```python
from build123d import *

# Parameters (mm, degrees)
CROQUIS1_R              = 4
SALIENTE_EXTRUIR1_DEPTH = 1.497272789
CROQUIS3_R              = 2.5
CORTAR_EXTRUIR2_DEPTH   = 3
CROQUIS4_R              = 15.8
CORTAR_EXTRUIR3_DEPTH   = 10
CROQUIS5_W              = 12
CROQUIS5_H              = 7.5
CORTAR_EXTRUIR4_DEPTH   = 10
CROQUIS6_R              = 1.600000002
CORTAR_EXTRUIR5_DEPTH   = 10
CROQUIS9_R              = 1.787352587
CROQUIS9_R_2            = 1.8
CROQUIS9_R_3            = 1.832705365
CROQUIS9_R_4            = 1.812354621
CORTAR_EXTRUIR7_DEPTH   = 10
CROQUIS10_R             = 2
CROQUIS10_R_2           = 2.1
CORTAR_EXTRUIR8_DEPTH   = 10


with BuildPart() as part:
    # Croquis1 → Saliente-Extruir1 (new, symmetric)
    with BuildSketch(Plane(origin=(0, 0, 0), x_dir=(1, 0, 0), z_dir=(0, 1, 0))):
        Polygon((-77, -42), (-77, -54), (77, -54), (77, -42), (74, -42), (74, -28), (77, -28), (77, -20), (74, -20), (74, -12), (77, -12), (77, -4), (74, -4), (74, -1.5), (74, 1.5), (74, 4), (77, 4), (77, 12), (74, 12), (74, 14.497912952), (70.25, 14.497912952), (70.25, 12), (67.25, 12), (67.25, 14.497912952), (66.27, 14.497912952), (66.27, 17.992083938), (67.25, 17.992083938), (67.25, 20), (70.25, 20), (70.25, 17.992083938), (74, 17.992083938), (74, 20), (77, 20), (77, 28), (74, 28), (74, 42), (77, 42), (77, 54), (65, 54), (65, 51), (55, 51), (55, 54), (45, 54), (45, 51), (31.5, 51), (31.5, 47.25), (34, 47.25), (34, 44.25), (31.5, 44.25), (31.5, 43.27), (28.5, 43.27), (28.5, 44.25), (26, 44.25), (26, 47.25), (28.5, 47.25), (28.5, 51), (15, 51), (15, 54), (5, 54), (5, 51), (-5, 51), (-5, 54), (-15, 54), (-15, 51), (-28.5, 51), (-28.5, 47.25), (-26, 47.25), (-26, 44.25), (-28.5, 44.25), (-28.5, 43.27), (-31.5, 43.27), (-31.5, 44.25), (-34, 44.25), (-34, 47.25), (-31.5, 47.25), (-31.5, 51), (-45, 51), (-45, 54), (-55, 54), (-55, 51), (-65, 51), (-65, 54), (-77, 54), (-77, 42), (-74, 42), (-74, 28), (-77, 28), (-77, 20), (-74, 20), (-74, 17.992083938), (-70.25, 17.992083938), (-70.25, 20), (-67.25, 20), (-67.25, 17.992083938), (-66.27, 17.992083938), (-66.27, 14.497912952), (-67.25, 14.497912952), (-67.25, 12), (-70.25, 12), (-70.25, 14.497912952), (-74, 14.497912952), (-74, 12), (-77, 12), (-77, 4), (-74, 4), (-74, 1.5), (-74, -1.5), (-74, -4), (-77, -4), (-77, -12), (-74, -12), (-74, -20), (-77, -20), (-77, -28), (-74, -28), (-74, -42), align=None)
        with Locations(Location((-65, -48, 0), (0, 0, 270))):
            Circle(CROQUIS1_R, mode=Mode.SUBTRACT)
        with BuildLine():
            Line((55, -49.6), (53, -49.6))
            ThreePointArc((53, -49.6), (52.646446609, -49.453553391), (52.5, -49.1))
            Line((52.5, -49.1), (52.5, -46.4))
            Line((52.5, -46.4), (55.5, -46.4))
            Line((55.5, -46.4), (55.5, -49.1))
            ThreePointArc((55.5, -49.1), (55.353553391, -49.453553391), (55, -49.6))
        make_face(mode=Mode.SUBTRACT)
    extrude(amount=SALIENTE_EXTRUIR1_DEPTH, both=True)

    # Croquis3 → Cortar-Extruir2 (cut)
    with BuildSketch(Plane(origin=(0, 1.497272789, 0), x_dir=(1, 0, 0), z_dir=(0, 1, 0))):
        with Locations(Location((-19.5, 33.79, 0), (0, 0, 270))):
            Circle(CROQUIS3_R)
        with Locations(Location((19.5, 33.79, 0), (0, 0, 270))):
            Circle(CROQUIS3_R)
    extrude(amount=-CORTAR_EXTRUIR2_DEPTH, mode=Mode.SUBTRACT)

    # Croquis4 → Cortar-Extruir3 (cut)
    with BuildSketch(Plane.XZ.offset(1.497272789)):
        with Locations(Location((0, -33.79, 0), (0, 0, 270))):
            Circle(CROQUIS4_R)
    extrude(amount=-CORTAR_EXTRUIR3_DEPTH, mode=Mode.SUBTRACT)

    # Croquis5 → Cortar-Extruir4 (cut)
    with BuildSketch(Plane.XZ.offset(1.497272789)):
        with Locations((-33.25, -35.6)):
            Rectangle(CROQUIS5_W, CROQUIS5_H)
        with Locations((33.25, -35.6)):
            Rectangle(CROQUIS5_W, CROQUIS5_H)
    extrude(amount=-CORTAR_EXTRUIR4_DEPTH, mode=Mode.SUBTRACT)

    # Croquis6 → Cortar-Extruir5 (cut)
    with BuildSketch(Plane(origin=(0, 1.497272789, 0), x_dir=(1, 0, 0), z_dir=(0, 1, 0))):
        with Locations(Location((33.25, 13.2, 0), (0, 0, 270))):
            Circle(CROQUIS6_R)
        with Locations(Location((-33.25, 13.2, 0), (0, 0, 270))):
            Circle(CROQUIS6_R)
    extrude(amount=-CORTAR_EXTRUIR5_DEPTH, mode=Mode.SUBTRACT)

    # Croquis9 → Cortar-Extruir7 (cut)
    with BuildSketch(Plane(origin=(0, 1.497272789, 0), x_dir=(1, 0, 0), z_dir=(0, 1, 0))):
        with Locations(Location((69.85, 46.119647413, 0), (0, 0, 270))):
            Circle(CROQUIS9_R)
        with Locations(Location((69.8, 27.693127607, 0), (0, 0, 270))):
            Circle(CROQUIS9_R_2)
        with Locations(Location((69.85, -21.925705365, 0), (0, 0, 270))):
            Circle(CROQUIS9_R_3)
        with Locations(Location((69.8, -40.306872393, 0), (0, 0, 270))):
            Circle(CROQUIS9_R_2)
        with Locations(Location((-69.8, -40.306872393, 0), (0, 0, 270))):
            Circle(CROQUIS9_R_2)
        with Locations(Location((-69.85, -21.925705365, 0), (0, 0, 270))):
            Circle(CROQUIS9_R_3)
        with Locations(Location((-66.4, 27.693127607, 0), (0, 0, 270))):
            Circle(CROQUIS9_R_2)
        with Locations(Location((-66.4, 46.119647413, 0), (0, 0, 270))):
            Circle(CROQUIS9_R_4)
    extrude(amount=-CORTAR_EXTRUIR7_DEPTH, mode=Mode.SUBTRACT)

    # Croquis10 → Cortar-Extruir8 (cut)
    with BuildSketch(Plane(origin=(0, 1.497272789, 0), x_dir=(1, 0, 0), z_dir=(0, 1, 0))):
        with Locations(Location((-19, 4.95, 0), (0, 0, 270))):
            Circle(CROQUIS10_R)
        with Locations(Location((19, 4.95, 0), (0, 0, 270))):
            Circle(CROQUIS10_R_2)
        with Locations(Location((19, -33.05, 0), (0, 0, 270))):
            Circle(CROQUIS10_R_2)
        with Locations(Location((-19, -33.05, 0), (0, 0, 270))):
            Circle(CROQUIS10_R)
    extrude(amount=-CORTAR_EXTRUIR8_DEPTH, mode=Mode.SUBTRACT)


solid = part.part
```
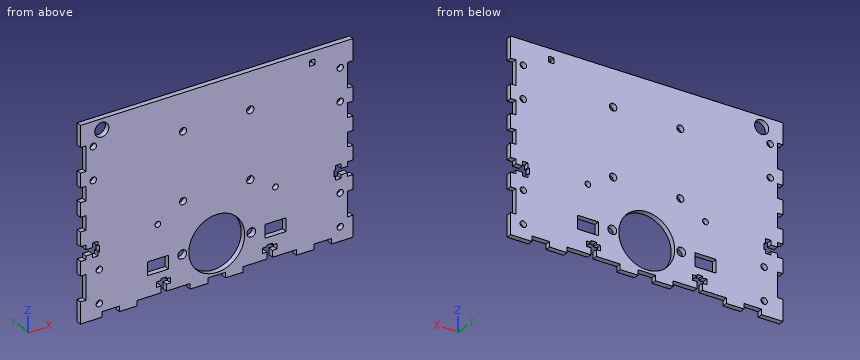
Model file for the job. Use its own axes, mm. Coordinates: 2 decimals unless noted, no trailing zeros. Loops run counter-clockwise (first coordinate to the right, second up) from the corner with the lowest first, then second, coordinate; pieces in that order, holes last. Notation, with made-up numbers: M 36.5,20 L 69.5,20 A22 cw 69.5,42 Z; hole C -9.75,71.5 d11. An arc over 180 degrees is marked long. Use CSV: the item, a comma, the result in double quotes. Start each with the question number.
1. Band-saw the part on A-A, the plane y = -0.1. Give the number of separate pieces and of enclosed holes in the cut face, then the cut area to 3 significant figures.
2. Probe probe 1 along X at (y, z) = (-0.1, -33.79); probe 2 along Z at (x, y) = (70, 1); probe 3 along X at (y, z) = (-0.25, -4.95). List the from-to ranges inside material, lowest first. Write a range as [from, to].
3. Band-saw the part on B-B, the plane x = 62. List the corners of the cut face in (y, z), then the cut area to 3 significant figures.
4. Flat gauge pins, fed straight in: pin 1 (1.5 mm diameter, centred on y = -0.5, z = -35, fed in from -X); pin 2 (1.6 mm diameter, centred on y = 0.5, z = -19, fed in from +X). Where does each tip first touch, or does it go through?
Entries:
1,separate pieces,"1"
1,enclosed holes,"21"
1,area,"14,700 mm2"
2,probe 1,"x = [-74, -39.25], [-27.25, -22], [-17, -15.8], [15.8, 17], [22, 27.25], [39.25, 74]"
2,probe 2,"z = [-54, -47.9], [-44.34, -29.48], [-25.9, -20], [-12, 20.1], [23.75, 38.52], [42.1, 54]"
2,probe 3,"x = [-77, -21], [-17, 16.9], [21.1, 77]"
3,outline,"M -1.5,-51 L 1.5,-51 L 1.5,54 L -1.5,54 Z"
3,area,"314 mm2"
4,pin 1,"stops at x = -74"
4,pin 2,"stops at x = 74"
